Part model, mm, in its own coordinate system. Face numbers are marked on the shaded views. A direction names the side the tool comes from. Round coordinates to 2 decimals unless told otherwise and drop trailing zeros. Write each loop counter-clockwise with the first axis right and the second up, starting at its lowest first coordinate (ties: lowest second). Pieces come first, ordered by that corner, then holes. Notation, with made-up numbers: M 5.5,-22 L 17.5,-22 A19 ccw 17.5,-9 Z; hole C -31,72 d8. An arc over 180 degrees is marked long. One line per question, with ' | ' between items. Start each with the question number.
1) Saw through at C-C (y = -0.95). List the corners of the cut face in (x, z).
2) Wall check: probe 1 along Z at (x, y) = (0, -3.3); probe 2 along Z at (x, y) = (0, -1.65); probe 3 along X at (y, z) = (-4.4, -0.5). Give the ranges that are in metal, low to high. Write a range as [from, to].
3) Saw through at A-A (x = 0). List the corners of the cut face in (y, z), plus the area to 3 significant figures.
4) Drop flat-ended pins along their axis: pin 1 Ø2 at (x, z) = (-2, 1.5) entering from +Y; pin 2 Ø1.5 at (x, y) = (1.5, -3) entering from -Z. Give the stop position or say it passes through.
5) Tool access for the marked faces 4 and 5: list every direction of +Z, -Z, +X, -X, +Y, -Y with a clear straight run to the whole face (end or side of a thin tool).
6) Mould opens along X. For the marked faces 1, 2 and 3 say: pulls with the +X half, pulls with the -X half, needs draft (parallel to the pull), parting line crosses it, or undercut.
7) Saw through at B-B (z = 0). List the corners of the cut face in (x, y), plus the area to 3 significant figures.
8) Saw through at D-D (y = -3.25). List the corners of the cut face in (x, z).
```python
from build123d import *

# Parameters (mm, degrees)
CHAMFER1_SIZE = 0.254


with BuildPart() as part:
    # Sketch1 → Revolve1 (revolve)
    with BuildSketch(Plane.XY):
        Polygon((5.016, 0), (5.016, -2.54), (6, -2.54), (6, -4.572), (4, -4.572), (4, 0), align=None)
    revolve(axis=Axis((0, 0, 0), (0, -1, 0)))

    # Chamfer1
    chamfer1_edges = [part.edges().sort_by_distance(p)[0] for p in [
        (-6, -4.572, 0),
        (-6, -2.54, 0),
        (-5.016, 0, 0),
    ]]
    chamfer(chamfer1_edges, length=CHAMFER1_SIZE)


solid = part.part
```
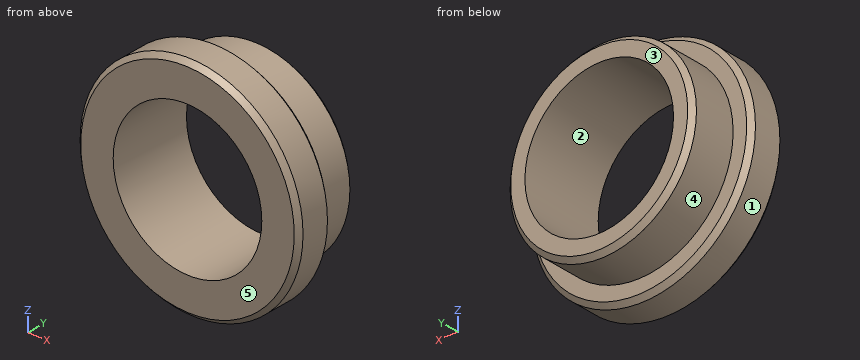
Answer key:
1) outline: C 0,0 d10.03; hole C 0,0 d8
2) probe 1: z = [-6, -4], [4, 6] | probe 2: z = [-5.02, -4], [4, 5.02] | probe 3: x = [-5.9, -3.97], [3.97, 5.9]
3) outline: M -4.57,-5.75 L -4.32,-6 L -2.79,-6 L -2.54,-5.75 L -2.54,-5.02 L -0.25,-5.02 L 0,-4.76 L 0,-4 L -4.57,-4 Z; M -4.57,4 L 0,4 L 0,4.76 L -0.25,5.02 L -2.54,5.02 L -2.54,5.75 L -2.79,6 L -4.32,6 L -4.57,5.75 Z | area: 13.1 mm2
4) pin 1: passes through | pin 2: stops at z = -5.95
5) face 4: +Y | face 5: +Z, -Z, +X, -X, -Y
6) face 1: parting line crosses it | face 2: undercut | face 3: needs draft
7) outline: M -6,-4.32 L -5.75,-4.57 L -4,-4.57 L -4,0 L -4.76,0 L -5.02,-0.25 L -5.02,-2.54 L -5.75,-2.54 L -6,-2.79 Z; M 4,-4.57 L 5.75,-4.57 L 6,-4.32 L 6,-2.79 L 5.75,-2.54 L 5.02,-2.54 L 5.02,-0.25 L 4.76,0 L 4,0 Z | area: 13.1 mm2
8) outline: C 0,0 d12; hole C 0,0 d8
